Geometry check sheet. Reference: the model listing, model coordinates, mm. Face numbers are marked on the shaded views. A direction names the side the tool comes from. Give positions to 0.01 mm unless a question says otherwise; leave off trailing zeros. Loops run counter-clockwise (first coordinate to the right, second up) from the corner with the lowest first, then second, coordinate; pieces in that order, holes last. Notation, with made-up numbers: (47.25, -25) -> (76.25, -25) arc R10 cw to (76.25, -11) -> close; hole circle Ø11 at (15.5, 10.5). An arc over 180 degrees is marked (long way). Write each question's results on one line, items separated by ' | '. Start each with the question number.
1) Draft check along Z on the marked faces 1, 2 and 3. Enter one of: pulls with the +Z half, pulls with the -Z half, needs draft (parallel to the pull), parting line crosses it, or undercut.
2) Sectioned sample at C-C on y = 83. Record the cut outline in (x, z).
3) Scan lines: line 1 (Z direction, x = 8.5, y = 94.5); line 2 (Y direction, x = -29, z = 14.5). Record each from-to range of solid material in increasing order. Write a range as from..to.
4) Set-up check for the marked faces 4, 5 and 6: record each of +Z, -Z, +X, -X, +Y, -Y from which the full face is reachable in a straight line by a thin tool's end or side.
5) Sectioned sample at A-A on x = 0. Record the cut outline in (y, z).
6) Sectioned sample at D-D on z = 33. Record the cut outline in (x, y).
7) Sectioned sample at B-B on z = 0. Record the cut outline in (x, y), then the cut area to 3 significant figures.
8) Depth check by flat-ended pin: pin 1 (1.5 mm diameter, centred on y = 1, z = -63, fed in from -X); pin 2 (5.5 mm diameter, centred on y = -2, z = 62.5, fed in from +X); pin 3 (8 mm diameter, centred on x = -15.5, y = 83, fed in from +Z). Enter the tip coordinate at first touch or a pass-through.
```python
from build123d import *

# Parameters (mm, degrees)
SKETCH1_W           = 100
SKETCH1_H           = 100
SKETCH1_W_2         = 80
SKETCH1_H_2         = 80
BOSS_EXTRUDE1_DEPTH = 140
SKETCH2_W           = 100
SKETCH2_H           = 100
SKETCH2_R           = 25
BOSS_EXTRUDE2_DEPTH = 5
SKETCH3_W           = 40
SKETCH3_H           = 25
BOSS_EXTRUDE3_DEPTH = 10
SKETCH4_R           = 3
CUT_EXTRUDE1_DEPTH  = 10
FILLET1_R           = 10


with BuildPart() as part:
    # Sketch1 → Boss-Extrude1 (new body)
    with BuildSketch(Plane(origin=(0, 0, 0), x_dir=(1, 0, 0), z_dir=(0, 1, 0))):
        Rectangle(SKETCH1_W, SKETCH1_H)
        Rectangle(SKETCH1_W_2, SKETCH1_H_2, mode=Mode.SUBTRACT)
    extrude(amount=BOSS_EXTRUDE1_DEPTH)

    # Sketch2 → Boss-Extrude2 (add)
    with BuildSketch(Plane.XZ):
        Rectangle(SKETCH2_W, SKETCH2_H)
        with Locations(Location((0, 0, 0), (0, 0, 270))):
            Circle(SKETCH2_R, mode=Mode.SUBTRACT)
    extrude(amount=BOSS_EXTRUDE2_DEPTH)

    # Sketch3 → Boss-Extrude3 (add)
    with BuildSketch(Plane.XZ.offset(5)):
        with Locations((0, 62.5)):
            Rectangle(SKETCH3_W, SKETCH3_H)
        with Locations((0, -62.5)):
            Rectangle(SKETCH3_W, SKETCH3_H)
    extrude(amount=-BOSS_EXTRUDE3_DEPTH)

    # Sketch4 → Cut-Extrude1 (cut)
    with BuildSketch(Plane(origin=(0, 5, 0), x_dir=(1, 0, 0), z_dir=(0, 1, 0))):
        with Locations(Location((0, 67, 0), (0, 0, 270))):
            Circle(SKETCH4_R)
        with Locations(Location((0, -67, 0), (0, 0, 90))):
            Circle(SKETCH4_R)
    extrude(amount=-CUT_EXTRUDE1_DEPTH, mode=Mode.SUBTRACT)

    # Fillet1
    fillet1_edges = [part.edges().sort_by_distance(p)[0] for p in [
        (-20, 0, 50),
        (-20, 0, 75),
        (20, 0, 75),
        (20, 0, 50),
        (-20, 0, -50),
        (20, 0, -50),
        (20, 0, -75),
        (-20, 0, -75),
    ]]
    fillet(fillet1_edges, radius=FILLET1_R)


solid = part.part
```
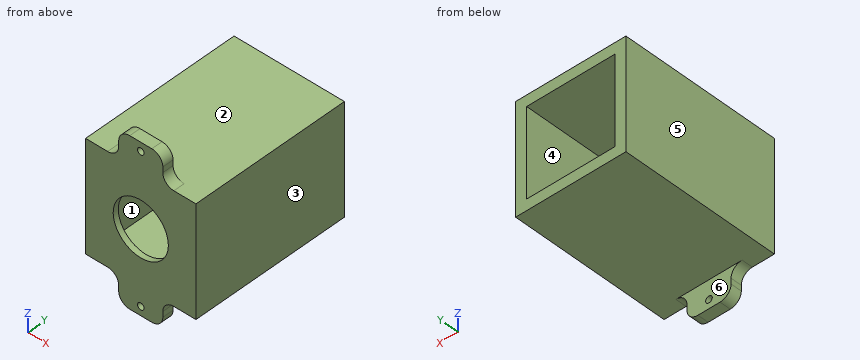
Result:
1) face 1: undercut | face 2: pulls with the +Z half | face 3: needs draft
2) outline: (-50, -50) -> (50, -50) -> (50, 50) -> (-50, 50) -> close; hole (-40, -40) -> (40, -40) -> (40, 40) -> (-40, 40) -> close
3) line 1: -50..-40, 40..50 | line 2: -5..0
4) face 4: +Y | face 5: +Z, -Z, -X, +Y, -Y | face 6: -Z, +X, -X, +Y
5) outline: (-5, -75) -> (5, -75) -> (5, -70) -> (-5, -70) -> close; (-5, -64) -> (5, -64) -> (5, -50) -> (140, -50) -> (140, -40) -> (0, -40) -> (0, -25) -> (-5, -25) -> close; (-5, 25) -> (0, 25) -> (0, 40) -> (140, 40) -> (140, 50) -> (5, 50) -> (5, 64) -> (-5, 64) -> close; (-5, 70) -> (5, 70) -> (5, 75) -> (-5, 75) -> close
6) outline: (-50, -5) -> (50, -5) -> (50, 140) -> (40, 140) -> (40, 0) -> (-40, 0) -> (-40, 140) -> (-50, 140) -> close
7) outline: (-50, -5) -> (-25, -5) -> (-25, 0) -> (-40, 0) -> (-40, 140) -> (-50, 140) -> close; (25, -5) -> (50, -5) -> (50, 140) -> (40, 140) -> (40, 0) -> (25, 0) -> close | area: 3,050 mm^2
8) pin 1: x = -20 | pin 2: x = 20 | pin 3: z = 50
